The listing builds one solid part. Answer for the finished solid, in the listing's coordinates (mm). A direction names the side the tool comes from. Round coordinates to 2 decimals unless told otherwise and drop trailing zeros. Write each loop counter-clockwise with the first axis right and the second up, starting at its lowest first coordinate (ties: lowest second). Pieces come first, ordered by that corner, then holes.
(1) A cutting plane is placed at A-A, the plane z = 49. Give the vertices of the cut face in (x, y) (3 decimals).
(2) For faces 4 (the face through (5, 5, 6.35)), 5 (the face through (28, 18, 25.4)), 6 (the face through (27.715, -21.251, 16.79)), determine the directions among +Z, -Z, +X, -X, +Y, -Y from which every point of the face is accessible in a straight line to the end or side of a thin tool.
(3) Each of these flat-tipped pins is pushed along its axis until it touches: pin 1 Ø3 at (x, y) = (4.5, -16.5) entering from -Z; pin 2 Ø1 at (x, y) = (-14, 22) entering from +Z; pin 3 Ø2 at (y, z) = (-25.5, 147.5) entering from +X. Where does it stop, or does it pass through?
(4) Find the intervals of material crossed by probe 1 along Z at (x, y) = (-6, 12.5) (3 decimals); probe 2 along Y at (x, z) = (0, 170) (3 decimals); probe 3 along Y at (x, z) = (0, 5.25) (3 decimals), in increasing order.
(5) The mould has two halves that part along Y. Classify faces 1 (the face through (-0.2, 3.5, 0)), 2 (the face through (-4.92, -4.84, 303.57)), 3 (the face through (-10.764, -9.871, 303.486)): +Y half, -Y half, draft (parallel to the pull), parting line (faces both ways), or undercut.
Autodesk Inventor part; units mm, degrees
ref_plane "YZ Plane" through (0, 0, 0) normal (1, 0, 0) x (0, 1, 0)
ref_plane "XZ Plane" through (0, 0, 0) normal (0, 1, 0) x (-1, 0, 0)
ref_plane "XY Plane" through (0, 0, 0) normal (0, 0, 1) x (1, 0, 0)
sketch "Sketch1" plane through (0, 0, 0) normal (0, 0, 1) x (1, 0, 0)
  circle A0 centre (0, 0) radius 14.605
  dimension "d0" = 29.21
extrude "Extrusion1" add sketch "Sketch1" along normal blind 306.705
sketch "Sketch3" plane through (0, 0, 0) normal (0, 0, -1) x (-1, 0, 0)
  circle A0 centre (0, 0) radius 34.925
  circle A1 centre (0, 0) radius 14.605
  dimension "d4" = 69.85
extrude "Extrusion2" add sketch "Sketch3" against normal blind 25.4 contours A0 | A1
extrude "Extrusion3" cut sketch "Sketch3" against normal blind 8.382
sketch "Sketch4" plane through (0, 0, 25.4) normal (0, 0, 1) x (1, 0, 0)
  circle A0 centre (0, 0) radius 32.385
  dimension "d9" = 64.77
extrude "Extrusion4" add sketch "Sketch4" along normal blind 272.923
fillet "Fillet1" radius 1.27 3 edges at (34.925, 0, 25.4) (34.925, 0, 8.382) (-32.385, 0, 298.323)
sketch "Sketch5" plane through (0, 0, 0) normal (1, 0, 0) x (0, 1, 0)
  line L0 (-14.605, 0) -> (14.605, 0)
  line L1 (14.605, 0) -> (14.605, 6.35)
  line L2 (14.605, 8.382) -> (14.605, 0)
  line L3 (33.655, 8.382) -> (-33.655, 8.382)
  line L4 (14.605, 6.35) -> (33.655, 8.382)
  line L5 (0, -61.341) -> (0, 368.046)
  point P0 (0, 0)
  dimension "d13" = 6.35
revolve "Revolution1" add sketch "Sketch5" angle 360 about axis through (0, 0, -10) along (0, 0, 1) contours L2 L3 L4
sketch "Sketch6" plane through (0, 0, 0) normal (0, 1, 0) x (-1, 0, 0)
  line L0 (14.605, 306.705) -> (-14.605, 306.705)
  line L1 (14.605, 306.705) -> (14.605, 300.355)
  line L2 (14.605, 298.323) -> (14.605, 306.705)
  line L3 (14.605, 300.355) -> (31.115, 298.323)
  arc A0 (32.385, 297.053) -> (31.115, 298.323) centre (31.115, 297.053) ccw
  line L4 (14.605, 298.323) -> (-14.605, 298.323)
  line L5 (14.605, 306.705) -> (-14.605, 306.705)
  line L6 (-31.115, 298.323) -> (31.115, 298.323)
  line L7 (0, -61.341) -> (0, 368.046)
  point P0 (0, 0)
  dimension "d15" = 6.35
revolve "Revolution2" add sketch "Sketch6" angle 360 about axis through (0, 0, -10) along (0, 0, 1) contours L3 L6 L2
sketch "Sketch7" plane through (0, 0, 0) normal (0, 0, -1) x (-1, 0, 0)
  circle A0 centre (0, 0) radius 14.605
  circle A1 centre (0, 0) radius 3.175
  circle A2 centre (0, 0) radius 9.525
  line L0 (3.175, 0) -> (9.525, 0)
  line L1 (0, -3.175) -> (0, -9.525)
  line L2 (9.525, 0) -> (7.62, 0)
  line L3 (0, -9.525) -> (0, -7.62)
  line L4 (0, -7.62) -> (1.905, -7.62)
  line L5 (1.905, -7.62) -> (1.905, -5.715)
  line L6 (7.62, 0) -> (7.62, -1.905)
  line L7 (7.62, -1.905) -> (5.715, -1.905)
  arc A3 (1.905, -7.62) -> (7.62, -1.905) centre (0, 0) ccw construction
  arc A4 (2.136, -8.5441) -> (8.5441, -2.136) centre (0, 0) ccw
  arc A5 (1.674, -6.6959) -> (6.6959, -1.674) centre (0, 0) ccw
  arc A6 (1.674, -6.6959) -> (2.136, -8.5441) centre (1.905, -7.62) ccw
  arc A7 (8.5441, -2.136) -> (6.6959, -1.674) centre (7.62, -1.905) ccw
  dimension "d17" = 6.35
  dimension "d18" = 19.05
  dimension "d19" = 1.905
  dimension "d20" = 1.905
  dimension "d21" = 1.905
  dimension "d22" = 1.905
  dimension "d23" = 1.905
extrude "Extrusion5" cut sketch "Sketch7" against normal blind 6.35 contours A7 A4 A6 L4 L5 A5 L7 L6 | L6 L7 A5 A7 | A6 A5 L5 L4
pattern_circular "Circular Pattern1" count 4 over 360 about axis through (0, 0, -10) along (0, 0, 1) of "Extrusion5"
sketch "Sketch8" plane through (0, 0, 0) normal (0, 0, -1) x (-1, 0, 0)
  circle A0 centre (0, 0) radius 6.35
  dimension "d29" = 12.7
sketch "Sketch9" plane through (0, 0, 25.4) normal (0, 0, 1) x (1, 0, 0)
  circle A0 centre (0, 0) radius 3.2385
  circle A1 centre (0, 0) radius 31.75
  dimension "d30" = 6.477
  dimension "d31" = 63.5
extrude "Extrusion6" cut sketch "Sketch9" along normal blind 271.653 contours A0 | A1
sketch "Sketch10" plane through (0, 0, 0) normal (0, 0, -1) x (-1, 0, 0)
  circle A0 centre (0, 0) radius 3.175
  dimension "d34" = 6.35
extrude "Extrusion7" cut sketch "Sketch10" along normal through all both and the other way through all
extrude "Extrusion8" cut sketch "Sketch9" against normal blind 15.24 contours A0 | A1
sketch "Sketch11" plane through (0, 0, 306.705) normal (0, 0, 1) x (1, 0, 0)
  circle A0 centre (0, 0) radius 14.605
  circle A1 centre (0, 0) radius 3.175
  circle A2 centre (0, 0) radius 9.525
  line L0 (3.175, 0) -> (9.525, 0)
  line L1 (0, -3.175) -> (0, -9.525)
  line L2 (9.525, 0) -> (7.62, 0)
  line L3 (0, -9.525) -> (0, -7.62)
  line L4 (0, -7.62) -> (1.905, -7.62)
  line L5 (1.905, -7.62) -> (1.905, -5.9372)
  line L6 (7.62, 0) -> (7.62, -1.905)
  line L7 (7.62, -1.905) -> (5.3447, -1.905)
  arc A3 (1.905, -7.62) -> (7.62, -1.905) centre (0, 0) ccw construction
  arc A4 (2.136, -8.5441) -> (8.5441, -2.136) centre (0, 0) ccw
  arc A5 (1.674, -6.6959) -> (6.6959, -1.674) centre (0, 0) ccw
  arc A6 (1.674, -6.6959) -> (2.136, -8.5441) centre (1.905, -7.62) ccw
  arc A7 (8.5441, -2.136) -> (6.6959, -1.674) centre (7.62, -1.905) ccw
  dimension "d39" = 6.35
  dimension "d40" = 19.05
  dimension "d41" = 1.905
  dimension "d42" = 1.905
  dimension "d43" = 1.905
  dimension "d44" = 1.905
  dimension "d45" = 1.905
extrude "Extrusion9" cut sketch "Sketch11" against normal blind 6.35 contours A7 A4 A6 L4 L5 A5 L7 L6 | L6 L7 A5 A7 | A6 A5 L5 L4
pattern_circular "Circular Pattern2" count 4 over 360 about axis through (0, 0, -10) along (0, 0, 1) of "Extrusion9"
properties part number "2.5X12inAirTank"
Solutions:
1. outline: circle Ø64.77 at (0, 0); hole circle Ø63.5 at (0, 0)
2. face 4: -Z
2. face 5: +Z
2. face 6: +Z, -Z
3. pin 1: stops at z = 6.46
3. pin 2: stops at z = 299
3. pin 3: stops at x = 21.18
4. probe 1: z = 0 to 10.16, 297.053 to 306.705
4. probe 2: y = -32.385 to -31.75, 31.75 to 32.385
4. probe 3: y = -14.605 to -3.175, 3.175 to 14.605
5. face 1: draft
5. face 2: undercut
5. face 3: parting line
